from build123d import *

# Parameters (mm, degrees)
SKETCH_W     = 15
SKETCH_H     = 50
SKETCH_R     = 2.75
PAD_DEPTH    = 3
PAD002_DEPTH = 10
SKETCH004_R  = 28.3
POCKET_DEPTH = 5
PAD003_DEPTH = 3
PAD004_DEPTH = 2


with BuildPart() as part:
    # Sketch → Pad (new body)
    with BuildSketch(Plane.XZ):
        with Locations((0, 15)):
            Rectangle(SKETCH_W, SKETCH_H)
        Circle(SKETCH_R, mode=Mode.SUBTRACT)
    extrude(amount=PAD_DEPTH)

    # Sketch003 → Pad002 (join)
    with BuildSketch(Plane.XZ):
        with BuildLine():
            ThreePointArc((26.676803, 47.276), (0, 91), (-26.676803, 47.276))
            Line((-26.676803, 47.276), (-7.5, 10))
            Line((-7.5, 10), (7.5, 10))
            Line((7.5, 10), (26.676803, 47.276))
        make_face()
    extrude(amount=PAD002_DEPTH)

    # Sketch004 (on DatumPlane) → Pocket (cut)
    with BuildSketch(Plane.XZ.offset(5)):
        with Locations((0, 61)):
            Circle(SKETCH004_R)
    extrude(amount=POCKET_DEPTH, mode=Mode.SUBTRACT)

    # Sketch006 (on DatumPlane) → Pad003 (join, symmetric)
    with BuildSketch(Plane.XY.offset(28)):
        with BuildLine():
            ThreePointArc((0, -10), (-2.828427, -11.171573), (-4, -14))
            Line((-4, -14), (-5, -14))
            Line((-5, -14), (-10, -10))
            Line((-10, -10), (0, -10))
        make_face()
    pad003 = extrude(amount=PAD003_DEPTH, both=True)

    # Mirrored: Pad003 across Sketch006 V_Axis
    add(pad003.mirror(Plane(origin=(0, 0, 28), x_dir=(0, 0, 1), z_dir=(1, 0, 0))))

    # Sketch007 (on DatumPlane) → Pad004 (join)
    with BuildSketch(Plane.YZ.offset(7.5)):
        Polygon((-3, -10), (-10, 10), (0, 10), (0, -10), align=None)
    pad004 = extrude(amount=-PAD004_DEPTH)

    # Mirrored001: Pad004 across YZ
    add(pad004.mirror(Plane.YZ))


solid = part.part
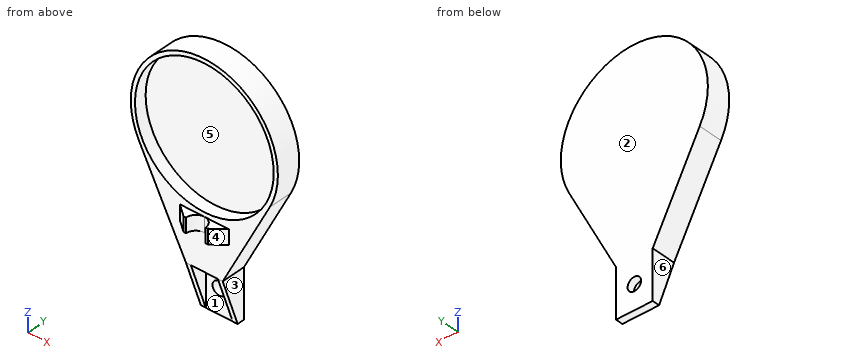
Source: CAD feature listing. Evaluate the final solid. Frame: model axes, mm. Face numbers are marked on the shaded views. A direction names the side the tool comes from. Coordinates: 2 decimals unless noted, no trailing zeros. Loops run counter-clockwise (first coordinate to the right, second up) from the corner with the lowest first, then second, coordinate; pieces in that order, holes last. Notation, with made-up numbers: (16, -31) - (50, -31) arc R19 cw to (50, 3) - close; hole circle Ø8 at (-12.75, 26.25). An arc over 180 degrees is marked (long way). One line per item, written item: value. Start each with the question number.
1. Section D-D (z = 30). Return the cut outline in (x, y), and give its area (3 significant figures).
2. Set-up query: the marked faces 1, 2 and 3. Return all of +Z, -Z, +X, -X, +Y, -Y with unobstructed straight access to the full face (end or side cutting, diameter ignored); none if empty.
3. Ray query, L1, parallel to Z at x = 0, y = -1.75; L2, parallel to Z at x = 0, y = -6.35; L3, parallel to X at y = -7.25, z = 84. Return the intervals inside material, ascending.
4. Section C-C (x = 22.5). Return the cut outline in (y, z), and give its area (3 significant figures).
5. Mould query, pull axis X, two halves, no side actions, for the marked faces 4, 5 and 6. Classes: pulls with the +X half, pulls with the -X half, needs draft (parallel to the pull), parting line crosses it, or undercut.
6. Contact query for flat-ended pins moving along their axis: P1, Ø3.5, axis at x = -0.5, y = -6.5, coming from the -Z side; P2, Ø7.5, axis at y = -5.5, z = 4, coming from the +X side; P3, Ø1.5, axis at y = -5, z = 75, coming from the -X side; P4, Ø1.2, axis at x = 3, y = -12.5, coming from the +Z side. Output: stop coordinate, or through.
7. Section A-A (z = 0). Return the cut outline in (x, y).
8. Section B-B (y = -8.25). Return the cut outline in (x, z), and give its area (3 significant figures).
Verdict:
1. outline: (-17.79, -10) - (-10, -10) - (-5, -14) - (-4, -14) arc R4 cw to (4, -14) - (5, -14) - (10, -10) - (17.79, -10) - (17.79, 0) - (-17.79, 0) - close
1. area: 391 mm2
2. face 1: -Z, -Y
2. face 2: +Z, -Z, +X, -X, +Y
2. face 3: -Z, +X, +Y, -Y
3. L1: z = -10 to -2.75, 2.75 to 91
3. L2: z = 10 to 32.7, 89.3 to 91
3. L3: x = -19.26 to -16.49, 16.49 to 19.26
4. outline: (-10, 39.16) - (0, 39.16) - (0, 80.84) - (-10, 80.84) - (-10, 78.17) - (-5, 78.17) - (-5, 43.83) - (-10, 43.83) - close
4. area: 245 mm2
5. face 4: pulls with the +X half
5. face 5: undercut
5. face 6: pulls with the -X half
6. P1: stops at z = 10
6. P2: stops at x = 7.5
6. P3: stops at x = -26.92
6. P4: passes through
7. outline: (-7.5, -6.5) - (-5.5, -6.5) - (-5.5, -3) - (-2.75, -3) - (-2.75, 0) - (-7.5, 0) - close; (2.75, -3) - (5.5, -3) - (5.5, -6.5) - (7.5, -6.5) - (7.5, 0) - (2.75, 0) - close
8. outline: (-26.68, 47.28) - (-7.5, 10) - (-7.5, 5) - (-5.5, 5) - (-5.5, 10) - (5.5, 10) - (5.5, 5) - (7.5, 5) - (7.5, 10) - (26.68, 47.28) arc R30 ccw (long way) to start; hole circle Ø56.6 at (0, 61)
8. area: 985 mm2
